Could you check a few things on this model? Use its own coordinates, in mm. Give positions to 0.01 mm unless a question says otherwise; leave off trailing zeros. Order: outer loops, then holes, each group sorted by start corner. A loop starts at its lowest first (then second) coordinate and runs counter-clockwise, first axis right, second up.
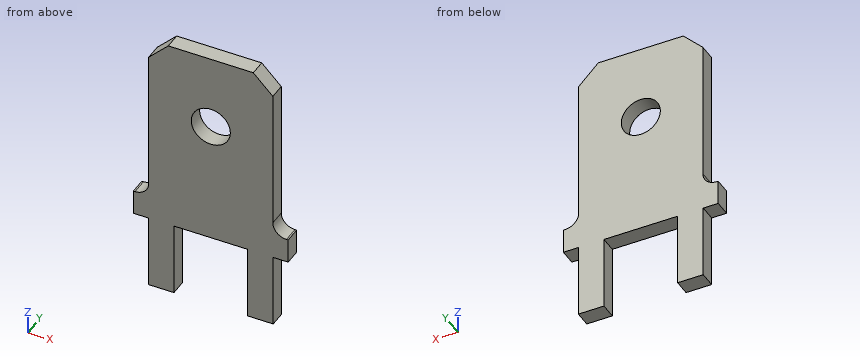
from build123d import *

# Parameters (mm, degrees)
F0_R     = 1
F1_DEPTH = 0.415
F2_SIZE  = 1
F3_R     = 0.7


with BuildPart() as f1:
    # F0 (on Front) → F1 (new body, symmetric)
    with BuildSketch(Plane.XZ):
        Polygon((-3.96, 1.27), (-3.96, 0), (-3.195, 0), (-3.195, -3.81), (-1.885, -3.81), (-1.885, 0), (1.885, 0), (1.885, -3.81), (3.195, -3.81), (3.195, 0), (3.96, 0), (3.96, 1.27), (3.175, 1.27), (3.175, 10.21), (-3.175, 10.21), (-3.175, 1.27), align=None)
        with Locations((0, 6.35)):
            Circle(F0_R, mode=Mode.SUBTRACT)
    extrude(amount=F1_DEPTH, both=True)

    # F2
    f2_edges = [f1.edges().sort_by_distance(p)[0] for p in [
        (3.175, 0, 10.21),
        (-3.175, 0, 10.21),
    ]]
    chamfer(f2_edges, length=F2_SIZE)

    # F3
    f3_edges = [f1.edges().sort_by_distance(p)[0] for p in [
        (3.175, 0, 1.27),
        (-3.175, 0, 1.27),
    ]]
    fillet(f3_edges, radius=F3_R)


solid = f1.part
Item 1: Imagine slicing it at D-D on z = 4. List the corners of the cut face in (x, y) for me (3 decimals), then the cut area to 3 significant figures.
Findings:
outline: (-3.175, -0.415) - (3.175, -0.415) - (3.175, 0.415) - (-3.175, 0.415) - close
area: 5.27 mm2
Item 2: Please list where these lines run through material, in increasing order: line 1 along X through (y, z) = (0.2, -0.75) (3 decimals); line 2 along Z through (x, y) = (0, -0.2); line 3 along Z through (x, y) = (-1.75, -0.3).
Findings:
line 1: x = -3.195 to -1.885, 1.885 to 3.195
line 2: z = 0 to 5.35, 7.35 to 10.21
line 3: z = 0 to 10.21
Item 3: Imagine slicing it at A-A on x = 0. List the corners of the cut face in (y, z) for me (3 decimals), then the cut area to 3 significant figures.
Findings:
outline: (-0.415, 0) - (0.415, 0) - (0.415, 5.35) - (-0.415, 5.35) - close; (-0.415, 7.35) - (0.415, 7.35) - (0.415, 10.21) - (-0.415, 10.21) - close
area: 6.81 mm2
Item 4: Imagine slicing it at B-B on z = 6.35. List the corners of the cut face in (x, y) for me (3 decimals), then the cut area to 3 significant figures.
Findings:
outline: (-3.175, -0.415) - (-1, -0.415) - (-1, 0.415) - (-3.175, 0.415) - close; (1, -0.415) - (3.175, -0.415) - (3.175, 0.415) - (1, 0.415) - close
area: 3.61 mm2
Item 5: Imagine slicing it at C-C on y = 0.2. List the corners of the cut face in (x, z) for me (3 decimals), then the cut area to 3 significant figures.
Findings:
outline: (-3.96, 0) - (-3.195, 0) - (-3.195, -3.81) - (-1.885, -3.81) - (-1.885, 0) - (1.885, 0) - (1.885, -3.81) - (3.195, -3.81) - (3.195, 0) - (3.96, 0) - (3.96, 1.27) - (3.875, 1.27) arc R0.7 cw to (3.175, 1.97) - (3.175, 9.21) - (2.175, 10.21) - (-2.175, 10.21) - (-3.175, 9.21) - (-3.175, 1.97) arc R0.7 cw to (-3.875, 1.27) - (-3.96, 1.27) - close; hole circle Ø2 at (0, 6.35)
area: 72.9 mm2
